from build123d import *

# Parameters (mm, degrees)
SKETCH1_W           = 80
SKETCH1_H           = 60
SKETCH1_R           = 1.55
BOSS_EXTRUDE1_DEPTH = 10
CUT_EXTRUDE1_REACH  = 52.99
SKETCH2_R           = 1.55
CUT_EXTRUDE2_REACH  = 52.99
SKETCH3_R           = 1.55


with BuildPart() as part:
    # Sketch1 → Boss-Extrude1 (new body)
    with BuildSketch(Plane.XY):
        Rectangle(SKETCH1_W, SKETCH1_H)
        with Locations((-20, 16)):
            Circle(SKETCH1_R, mode=Mode.SUBTRACT)
        with Locations((18, 16)):
            Circle(SKETCH1_R, mode=Mode.SUBTRACT)
        with Locations((18, -3)):
            Circle(SKETCH1_R, mode=Mode.SUBTRACT)
        with Locations((-20, -3)):
            Circle(SKETCH1_R, mode=Mode.SUBTRACT)
    extrude(amount=BOSS_EXTRUDE1_DEPTH)

    # Sketch2 → Cut-Extrude1 (cut, up to next)
    with BuildSketch(Plane(origin=(0, 0, 0), x_dir=(-1, 0, 0), z_dir=(0, 0, -1)), mode=Mode.PRIVATE) as cut_extrude1_sk1:
        with Locations((13, 26)):
            Circle(SKETCH2_R)
    cut_extrude1_tool1 = extrude(cut_extrude1_sk1.sketch, amount=-CUT_EXTRUDE1_REACH, mode=Mode.PRIVATE) & part.part
    add(cut_extrude1_tool1.solids().sort_by_distance((-13, 26, 0))[0], mode=Mode.SUBTRACT)

    # Sketch3 → Cut-Extrude2 (cut, up to next)
    with BuildSketch(Plane.XY.offset(10), mode=Mode.PRIVATE) as cut_extrude2_sk1:
        with Locations((32.5, 22)):
            Circle(SKETCH3_R)
    cut_extrude2_tool1 = extrude(cut_extrude2_sk1.sketch, amount=-CUT_EXTRUDE2_REACH, mode=Mode.PRIVATE) & part.part
    # Sketch3 → Cut-Extrude2 (cut, up to next)
    with BuildSketch(Plane.XY.offset(10), mode=Mode.PRIVATE) as cut_extrude2_sk2:
        with Locations((32.5, -22)):
            Circle(SKETCH3_R)
    cut_extrude2_tool2 = extrude(cut_extrude2_sk2.sketch, amount=-CUT_EXTRUDE2_REACH, mode=Mode.PRIVATE) & part.part
    add(cut_extrude2_tool1.solids().sort_by_distance((32.5, 22, 10))[0], mode=Mode.SUBTRACT)
    add(cut_extrude2_tool2.solids().sort_by_distance((32.5, -22, 10))[0], mode=Mode.SUBTRACT)


solid = part.part
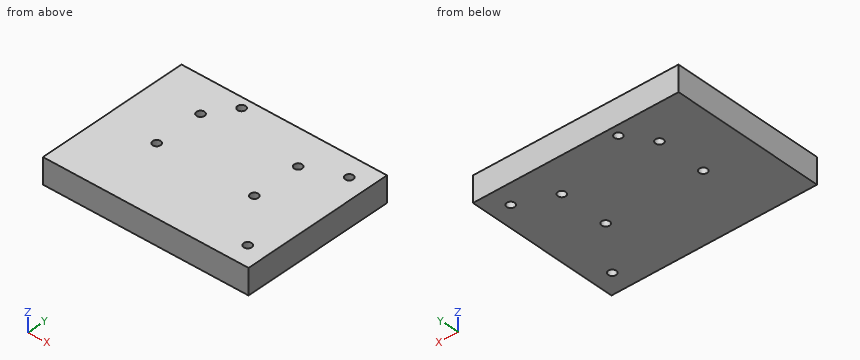
The model under review builds one solid part; all positions refer to its coordinate system, in mm. Round coordinates to 2 decimals unless told otherwise and drop trailing zeros. Loops run counter-clockwise (first coordinate to the right, second up) from the corner with the lowest first, then second, coordinate; pieces in that order, holes last. Notation, with made-up numbers: (23, -36) -> (36, -36) arc R28 cw to (36, -10) -> close; hole circle Ø7 at (88.25, -27). An arc over 180 degrees is marked (long way). Answer as CSV lines item,"result".
1) For P1, Ø2.5, axis at x = -20, y = -3, coming from the -Z side, flat-tipped, find the tip position at first contact; note if it passes through.
Geometry results:
P1,"passes through"
2) Add section C-C on y = 26. Write out the cut boundary in (x, z).
Geometry results:
outline,"(-40, 0) -> (-14.55, 0) -> (-14.55, 10) -> (-40, 10) -> close; (-11.45, 0) -> (40, 0) -> (40, 10) -> (-11.45, 10) -> close"
3) Add section B-B on y = 16. Write out the cut boundary in (x, z).
Geometry results:
outline,"(-40, 0) -> (-21.55, 0) -> (-21.55, 10) -> (-40, 10) -> close; (-18.45, 0) -> (16.45, 0) -> (16.45, 10) -> (-18.45, 10) -> close; (19.55, 0) -> (40, 0) -> (40, 10) -> (19.55, 10) -> close"
4) To check wall thickness, follow line 1 along Y through (x, z) = (-20, 5.25); line 2 along Y through (x, z) = (32.5, 7.5); line 3 along X through (y, z) = (17, 4.25). State the ranges of each line that lie inside material, in increasing order. Write a range as from..to.
Geometry results:
line 1,"y = -30..-4.55, -1.45..14.45, 17.55..30"
line 2,"y = -30..-23.55, -20.45..20.45, 23.55..30"
line 3,"x = -40..-21.18, -18.82..16.82, 19.18..40"
5) Add section A-A on x = -20. Write out the cut boundary in (y, z), plus the area to 3 significant figures.
Geometry results:
outline,"(-30, 0) -> (-4.55, 0) -> (-4.55, 10) -> (-30, 10) -> close; (-1.45, 0) -> (14.45, 0) -> (14.45, 10) -> (-1.45, 10) -> close; (17.55, 0) -> (30, 0) -> (30, 10) -> (17.55, 10) -> close"
area,"538 mm²"
